Work out the finished part from the listing and answer in its coordinate system (mm). Face numbers are marked on the shaded views. A direction names the side the tool comes from. Round coordinates to 2 decimals unless told otherwise and drop trailing zeros. Write each loop counter-clockwise with the first axis right and the second up, starting at its lowest first coordinate (ties: lowest second). Pieces come first, ordered by that corner, then holes. Notation, with made-up numbers: (-3.5, 8.25) -> (45.5, 8.25) arc R9 cw to (45.5, 23.25) -> close; hole circle Ø10 at (51, 24). An arc over 180 degrees is marked (long way). One line per item, written item: value.
Solid Edge part; units mm, degrees
sketch "Sketch1" plane through (0, 0, 0) normal (0, -1, 0) x (1, 0, 0)
  line L0 (57.5, -40.5) -> (57.5, 40.5)
  line L1 (57.5, 40.5) -> (-57.5, 40.5)
  line L2 (-57.5, 40.5) -> (-57.5, -40.5)
  line L3 (-57.5, -40.5) -> (57.5, -40.5)
extrude "Protrusion1" add sketch "Sketch1" along normal blind 31
sketch "Sketch2" plane through (0, 0, 0) normal (0, -1, 0) x (1, 0, 0)
  line L0 (-65.3, 23.5) -> (34.7, 23.5)
  line L1 (34.7, 23.5) -> (34.7, -30)
  line L2 (34.7, -30) -> (-65.3, -30)
  line L3 (-65.3, 23.5) -> (-65.3, -30)
extrude "Arduino" add sketch "Sketch2" against normal blind 16
sketch "Sketch3" plane through (0, 0, 0) normal (0, -1, 0) x (1, 0, 0)
  line L0 (-71.8, 14) -> (-71.8, 2.5)
  line L1 (-71.8, 2.5) -> (-57.5, 2.5)
  line L2 (-57.5, 2.5) -> (-57.5, 14)
  line L3 (-57.5, 14) -> (-65.3, 14)
  line L4 (-65.3, 14) -> (-71.8, 14)
  line L5 (-67.8, -18) -> (-67.8, -27)
  line L6 (-67.8, -27) -> (-57.5, -27)
  line L7 (-57.5, -27) -> (-57.5, -18)
  line L8 (-57.5, -18) -> (-64.65, -18)
  line L9 (-64.65, -18) -> (-67.8, -18)
extrude "Conectores" add sketch "Sketch3" against normal blind 16
sketch "Sketch4" plane through (0, 0, 0) normal (0, -1, 0) x (1, 0, 0)
  circle A0 centre (-50, 21) radius 1.5
  circle A1 centre (25, 21) radius 1.5
  circle A2 centre (31, -27.25) radius 1.5
  circle A3 centre (-51.25, -27) radius 1.5
  circle A4 centre (0.75, -22) radius 1.5
  circle A5 centre (0.75, 6) radius 1.5
extrude "Agujeros" cut sketch "Sketch4" along normal mid plane 70.2775
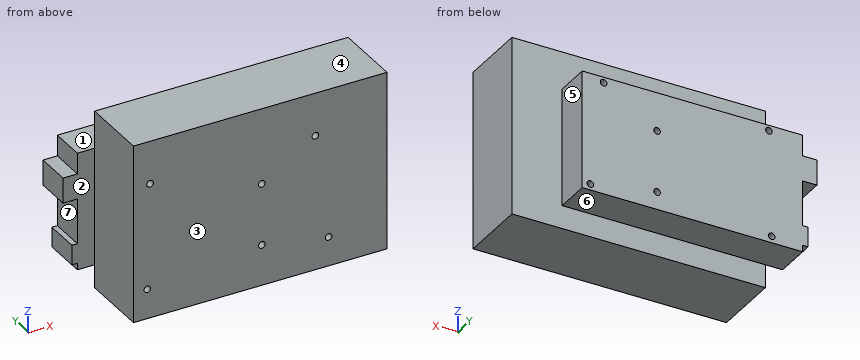
(1) Find section B-B on x = 25. Give the vertices of the cut face in (y, z), plus the area to 3 significant figures.
Reported:
outline: (-31, -40.5) -> (0, -40.5) -> (0, -30) -> (16, -30) -> (16, 19.5) -> (-31, 19.5) -> close; (-31, 22.5) -> (16, 22.5) -> (16, 23.5) -> (0, 23.5) -> (0, 40.5) -> (-31, 40.5) -> close
area: 3,230 mm2
(2) Consider probe 1 along X at (y, z) = (-10.5, 21); probe 2 along X at (y, z) = (6, -27.25); probe 3 along Z at (x, y) = (-50, 4.5). Determine where each line is inside the solid, lowest interval first.
Reported:
probe 1: x = -57.5 to -51.5, -48.5 to 23.5, 26.5 to 57.5
probe 2: x = -65.3 to -52.73, -49.77 to 29.5, 32.5 to 34.7
probe 3: z = -30 to -27.83, -26.17 to 19.5, 22.5 to 23.5
(3) Flat-ended cylindrical pins translate along their axes: pin 1 Ø6 at (y, z) = (0.5, 27.5) entering from +X; pin 2 Ø2.5 at (x, z) = (31, -27.25) entering from -Y; pin 3 Ø7 at (x, z) = (-63.5, 2) entering from -Y; pin 4 Ø3 at (x, y) = (-68.5, 8.5) entering from -Z. Find the tip coordinate at first contact, or state that the pin passes through.
Reported:
pin 1: stops at x = 57.5
pin 2: passes through
pin 3: stops at y = 0
pin 4: stops at z = -27
(4) For a pull along Z with two mould halves and no side action, classify the marked faces 4, 5, 6 and 7 as pulls with the +Z half, pulls with the -Z half, needs draft (parallel to the pull), parting line crosses it, or undercut.
Reported:
face 4: pulls with the +Z half
face 5: needs draft
face 6: pulls with the -Z half
face 7: undercut
(5) Find section C-C on y = 2. Give the vertices of the cut face in (x, z).
Reported:
outline: (-71.8, 2.5) -> (-65.3, 2.5) -> (-65.3, -18) -> (-67.8, -18) -> (-67.8, -27) -> (-65.3, -27) -> (-65.3, -30) -> (34.7, -30) -> (34.7, 23.5) -> (-65.3, 23.5) -> (-65.3, 14) -> (-71.8, 14) -> close; hole circle Ø3 at (-51.25, -27); hole circle Ø3 at (-50, 21); hole circle Ø3 at (0.75, -22); hole circle Ø3 at (0.75, 6); hole circle Ø3 at (25, 21); hole circle Ø3 at (31, -27.25)
(6) Find section A-A on z = 21. Give the vertices of the cut face in (x, y).
Reported:
outline: (-65.3, 0) -> (-57.5, 0) -> (-57.5, -31) -> (-51.5, -31) -> (-51.5, 16) -> (-65.3, 16) -> close; (-48.5, -31) -> (23.5, -31) -> (23.5, 16) -> (-48.5, 16) -> close; (26.5, -31) -> (57.5, -31) -> (57.5, 0) -> (34.7, 0) -> (34.7, 16) -> (26.5, 16) -> close
(7) A tool of negligible diameter and unlimited length cuts with its end or side. For the marked faces 1, 2 and 3, from which of +Z, -Z, +X, -X, +Y, -Y can it reach the whole face along a straight path? Write none if from no direction.
Reported:
face 1: +Z, +X, -X, +Y
face 2: +Z, -Z, -X, -Y
face 3: +Z, -Z, +X, -X, -Y
(8) Find section D-D on z = 6. Give the vertices of the cut face in (x, y), plus the area to 3 significant figures.
Reported:
outline: (-71.8, 0) -> (-57.5, 0) -> (-57.5, -31) -> (-0.75, -31) -> (-0.75, 16) -> (-71.8, 16) -> close; (2.25, -31) -> (57.5, -31) -> (57.5, 0) -> (34.7, 0) -> (34.7, 16) -> (2.25, 16) -> close
area: 5,130 mm2
